Autodesk Inventor part; units mm, degrees
ref_plane "YZ Plane" through (0, 0, 0) normal (1, 0, 0) x (0, 1, 0)
ref_plane "XZ Plane" through (0, 0, 0) normal (0, 1, 0) x (-1, 0, 0)
ref_plane "XY Plane" through (0, 0, 0) normal (0, 0, 1) x (1, 0, 0)
sketch "Sketch1" plane through (0, 0, 0) normal (0, 1, 0) x (-1, 0, 0)
  line L0 (-17.5, 10.1036) -> (0, 20.2073)
  line L1 (0, 20.2073) -> (17.5, 10.1036)
  line L2 (17.5, 10.1036) -> (17.5, -10.1036)
  line L3 (17.5, -10.1036) -> (0, -20.2073)
  line L4 (0, -20.2073) -> (-17.5, -10.1036)
  line L5 (-17.5, -10.1036) -> (-17.5, 10.1036)
  point P0 (0, 0)
  point P1 (0, 0)
  dimension "d0" = 35
extrude "Extrusion1" add sketch "Sketch1" along normal mid plane 20
sketch "Sketch2" plane through (0, 10, 0) normal (0, 1, 0) x (1, 0, 0)
  circle A0 centre (0, 0) radius 14.5
  dimension "d3" = 29
extrude "Extrusion2" cut sketch "Sketch2" against normal blind 18
chamfer "Chamfer1" distance 1 angle 80 1 edges at (-14.5, 10, 0) measured on face at (-8.579, 10, 14.0814)
Model file for the job. Use its own axes, mm. A direction names the side the tool comes from. Coordinates: 2 decimals unless noted, no trailing zeros. Loops run counter-clockwise (first coordinate to the right, second up) from the corner with the lowest first, then second, coordinate; pieces in that order, holes last. Notation, with made-up numbers: (-7, -6) -> (29, -6) arc R22 ccw to (29, 6) -> close; hole circle Ø2 at (32.5, 25.25). An arc over 180 degrees is marked (long way). Answer as a JSON object with one key per item and string values.
Q1. 3-axis set-ups, long thin cutter, end or side, ignore diameter. For faces 5 (the flat face through (8.628, -0.14, -15.226)), 6 (the cylindrical face through (6.691, -1.749, 12.864)): which of +Z, -Z, +X, -X, +Y, -Y reach the whole face in a straight line?
Report:
{"face 5": "-Z, +X, +Y, -Y", "face 6": "+Y"}
Q2. Probe probe 1 along Z at (x, y) = (0, -5); probe 2 along X at (y, z) = (-5.5, 0); probe 3 along Y at (x, z) = (9, -10.5). List the from-to ranges inside material, lowest first.
Report:
{"probe 1": "z = -20.21 to -14.5, 14.5 to 20.21", "probe 2": "x = -17.5 to -14.5, 14.5 to 17.5", "probe 3": "y = -10 to -8"}
Q3. Cut at A-A (y = -2.5). List the corners of the cut face in (x, z), and give its area (3 significant figures).
Report:
{"outline": "(-17.5, -10.1) -> (0, -20.21) -> (17.5, -10.1) -> (17.5, 10.1) -> (0, 20.21) -> (-17.5, 10.1) -> close; hole circle Ø29 at (0, 0)", "area": "400 mm2"}
Q4. Flat gauge pins, fed straight in: P1, Ø2, axis at x = 4, y = -1, coming from the +Z side; P2, Ø12, axis at x = 9.5, y = -2, coming from the -Z side; P3, Ø1.5, axis at y = -1.5, z = 11.5, coming from the -X side. Where does each tip first touch, or does it go through?
Report:
{"P1": "stops at z = 18.48", "P2": "stops at z = -18.19", "P3": "stops at x = -16.38"}
Q5. Cut at B-B (z = 0). List the corners of the cut face in (x, y).
Report:
{"outline": "(-17.5, -10) -> (17.5, -10) -> (17.5, 10) -> (15.5, 10) -> (14.5, 4.33) -> (14.5, -8) -> (-14.5, -8) -> (-14.5, 4.33) -> (-15.5, 10) -> (-17.5, 10) -> close"}
Q6. Pull direction Z, two halves, no side cores. Call faces 1 (the flat face through (0, -8, 0)), 2 (the flat face through (17.5, 0, 0)), 3 (the flat face through (-8.872, -0.14, -15.085)), 4 (the flat face through (-8.628, -0.14, 15.226)): released by +Z, released by -Z, zero draft, split by the parting line, or undercut.
Report:
{"face 1": "undercut", "face 2": "zero draft", "face 3": "released by -Z", "face 4": "released by +Z"}
Q7. Cut at C-C (y = 5). List the corners of the cut face in (x, z).
Report:
{"outline": "(-17.5, -10.1) -> (0, -20.21) -> (17.5, -10.1) -> (17.5, 10.1) -> (0, 20.21) -> (-17.5, 10.1) -> close; hole circle Ø29.24 at (0, 0)"}
